For this review, take the finished solid that the model builds, in its own axes (mm). Face numbers are marked on the shaded views. A direction names the side the tool comes from. Give positions to 0.01 mm unless a question says otherwise; leave off trailing zeros. Write each loop counter-clockwise with the first axis right and the second up, starting at its lowest first coordinate (ties: lowest second). Pieces come first, ordered by that corner, then holes. Notation, with made-up numbers: (70, -12) -> (123, -12) arc R29 cw to (123, 14) -> close; hole circle Ø9 at (-20, 6.5). An arc over 180 degrees is marked (long way). Write item = value, one per line.
```python
from build123d import *

# Parameters (mm, degrees)
SKETCH1_R           = 6
BOSS_EXTRUDE1_DEPTH = 100
SKETCH2_R           = 12.5
BOSS_EXTRUDE2_DEPTH = 20
SKETCH3_R           = 6
BOSS_EXTRUDE3_DEPTH = 20
SKETCH4_W           = 25
SKETCH4_H           = 14
BOSS_EXTRUDE4_DEPTH = 7
SKETCH5_W           = 25
SKETCH5_H           = 20
BOSS_EXTRUDE5_DEPTH = 7


with BuildPart() as part:
    # Sketch1 → Boss-Extrude1 (new body)
    with BuildSketch(Plane.XY):
        Circle(SKETCH1_R)
    extrude(amount=BOSS_EXTRUDE1_DEPTH)

    # Sketch2 → Boss-Extrude2 (add)
    with BuildSketch(Plane.XY.offset(100)):
        Circle(SKETCH2_R)
    extrude(amount=BOSS_EXTRUDE2_DEPTH)

    # Sketch3 → Boss-Extrude3 (add)
    with BuildSketch(Plane.XY.offset(120)):
        Circle(SKETCH3_R)
    extrude(amount=BOSS_EXTRUDE3_DEPTH)

    # Sketch4 → Boss-Extrude4 (add)
    with BuildSketch(Plane(origin=(0, 0, 0), x_dir=(-1, 0, 0), z_dir=(0, 0, -1))):
        Rectangle(SKETCH4_W, SKETCH4_H)
    extrude(amount=BOSS_EXTRUDE4_DEPTH)

    # Sketch5 → Boss-Extrude5 (add)
    with BuildSketch(Plane(origin=(0, 0, -7), x_dir=(-1, 0, 0), z_dir=(0, 0, -1))):
        Rectangle(SKETCH5_W, SKETCH5_H)
    extrude(amount=BOSS_EXTRUDE5_DEPTH)


solid = part.part
```
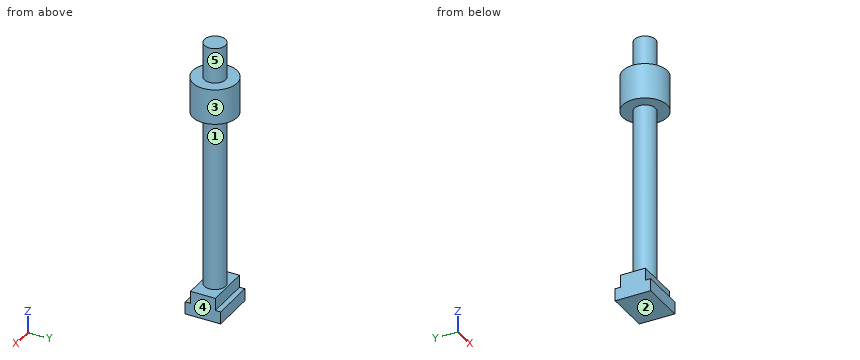
(1) Take a section at C-C (x = 0). Write out the cut boundary in (y, z), plus the area to 3 significant figures.
Answers below:
outline = (-12.5, 100) -> (-6, 100) -> (-6, 0) -> (-7, 0) -> (-7, -7) -> (-10, -7) -> (-10, -14) -> (10, -14) -> (10, -7) -> (7, -7) -> (7, 0) -> (6, 0) -> (6, 100) -> (12.5, 100) -> (12.5, 120) -> (6, 120) -> (6, 140) -> (-6, 140) -> (-6, 120) -> (-12.5, 120) -> close
area = 2,180 mm^2
(2) For pin 1 (8 mm diameter, centred on x = -6.5, z = 76.5, fed in from +Y); pin 2 (12 mm diameter, centred on x = -5.5, z = 49.5, fed in from -Y); pin 3 (5.5 mm diameter, centred on x = 2, z = -2, fed in from +Y), all flat-tipped, find the tip position at first contact; note any pin that passes through.
Answers below:
pin_1 = 5.45
pin_2 = -6
pin_3 = 7
(3) Take a section at A-A (x = 9). Write out the cut boundary in (y, z), plus the area to 3 significant figures.
Answers below:
outline = (-10, -14) -> (10, -14) -> (10, -7) -> (7, -7) -> (7, 0) -> (-7, 0) -> (-7, -7) -> (-10, -7) -> close; (-8.67, 100) -> (8.67, 100) -> (8.67, 120) -> (-8.67, 120) -> close
area = 585 mm^2
(4) Take a section at B-B (y = 8.5). Write out the cut boundary in (x, z), plus the area to 3 significant figures.
Answers below:
outline = (-12.5, -14) -> (12.5, -14) -> (12.5, -7) -> (-12.5, -7) -> close; (-9.17, 100) -> (9.17, 100) -> (9.17, 120) -> (-9.17, 120) -> close
area = 542 mm^2
(5) To check wall thickness, follow probe 1 along Z at (x, y) = (4.25, -5.25); probe 2 along Z at (x, y) = (-0.25, 9.25); probe 3 along X at (y, z) = (-0.5, 124). State the ranges of each line that lie inside material, in increasing order.
Answers below:
probe_1 = -14 to 0, 100 to 120
probe_2 = -14 to -7, 100 to 120
probe_3 = -5.98 to 5.98
(6) The part is to be moulded in two halves that separate along Z. For the marked faces 1, 2 and 3, say which applies: released by +Z, released by -Z, zero draft, split by the parting line, or undercut.
Answers below:
face_1 = undercut
face_2 = released by -Z
face_3 = zero draft
(7) Tool access review of the marked faces 4 and 5: name each direction out of +Z, -Z, +X, -X, +Y, -Y from which nothing blocks a thin tool from reaching the whole face with its end or side.
Answers below:
face_4 = +Z, -Z, +X, +Y, -Y
face_5 = +Z
(8) Take a section at D-D (y = 0). Write out the cut boundary in (x, z).
Answers below:
outline = (-12.5, -14) -> (12.5, -14) -> (12.5, 0) -> (6, 0) -> (6, 100) -> (12.5, 100) -> (12.5, 120) -> (6, 120) -> (6, 140) -> (-6, 140) -> (-6, 120) -> (-12.5, 120) -> (-12.5, 100) -> (-6, 100) -> (-6, 0) -> (-12.5, 0) -> close
